```python
from build123d import *

# Parameters (mm, degrees)
SKETCH1_R           = 6.35
BOSS_EXTRUDE1_DEPTH = 15.875
SKETCH2_R           = 7.9375
BOSS_EXTRUDE2_DEPTH = 22.225
BOSS_EXTRUDE3_START = 69.85
SKETCH3_R           = 6.35
BOSS_EXTRUDE3_DEPTH = 69.85
SKETCH4_R           = 6.35
BOSS_EXTRUDE4_DEPTH = 47.625
SKETCH5_OUTSIDE_W   = 52.458
SKETCH5_OUTSIDE_H   = 52.458
SKETCH5_OUTSIDE_R   = 6.223
CUT_EXTRUDE3_DEPTH  = 19.05
SKETCH6_OUTSIDE_W   = 52.458
SKETCH6_OUTSIDE_H   = 52.458
SKETCH6_OUTSIDE_R   = 6.223
CUT_EXTRUDE4_DEPTH  = 19.05


with BuildPart() as part:
    # Sketch1 → Boss-Extrude1 (new, symmetric)
    with BuildSketch(Plane(origin=(0, 0, 0), x_dir=(0, 0, -1), z_dir=(1, 0, 0))):
        Circle(SKETCH1_R)
    extrude(amount=BOSS_EXTRUDE1_DEPTH, both=True)

    # Sketch2 → Boss-Extrude2 (add)
    with BuildSketch(Plane.ZY.offset(15.875)):
        Circle(SKETCH2_R)
    extrude(amount=BOSS_EXTRUDE2_DEPTH)

    # Sketch3 → Boss-Extrude3 (add)
    with BuildSketch(Plane(origin=(15.875, 0, 0), x_dir=(0, 0, -1), z_dir=(1, 0, 0)).offset(BOSS_EXTRUDE3_START)):
        with Locations(Location((0, 0, 0), (0, 0, 180))):
            Circle(SKETCH3_R)
    extrude(amount=-BOSS_EXTRUDE3_DEPTH)

    # Sketch4 → Boss-Extrude4 (add)
    with BuildSketch(Plane.ZY.offset(38.1)):
        Circle(SKETCH4_R)
    extrude(amount=BOSS_EXTRUDE4_DEPTH)

    # Sketch5 outside → Cut-Extrude3 (cut)
    with BuildSketch(Plane.ZY.offset(85.725)):
        Rectangle(SKETCH5_OUTSIDE_W, SKETCH5_OUTSIDE_H)
        Circle(SKETCH5_OUTSIDE_R, mode=Mode.SUBTRACT)
    extrude(amount=-CUT_EXTRUDE3_DEPTH, mode=Mode.SUBTRACT)

    # Sketch6 outside → Cut-Extrude4 (cut)
    with BuildSketch(Plane(origin=(85.725, 0, 0), x_dir=(0, 0, -1), z_dir=(1, 0, 0))):
        Rectangle(SKETCH6_OUTSIDE_W, SKETCH6_OUTSIDE_H)
        with Locations(Location((0, 0, 0), (0, 0, 180))):
            Circle(SKETCH6_OUTSIDE_R, mode=Mode.SUBTRACT)
    extrude(amount=-CUT_EXTRUDE4_DEPTH, mode=Mode.SUBTRACT)


solid = part.part
```
Check sheet for the modelled part. Datum: model origin and axes. Units: mm. A direction names the side the tool comes from. Coordinates: 2 decimals unless noted, no trailing zeros. Loops run counter-clockwise (first coordinate to the right, second up) from the corner with the lowest first, then second, coordinate; pieces in that order, holes last.
1) Gauge pin test, flat ends, axial feed: pin 1 (6 mm diameter, centred on x = 20.5, y = 6, fed in from +Z); pin 2 (1 mm diameter, centred on x = -14, z = -2.5, fed in from -Y); pin 3 (1 mm diameter, centred on x = -41, z = 0.5, fed in from -Y). Record the tip position at first contact, or that the pin passes through.
2) Access from +Z, -Z, +X, -X, +Y, -Y to the whole of each face (thin tool, end or side, straight path). Record for faces 1 (the face through (-76.333, -6.075, -1.349)), 2 (the face through (-15.875, 7, 0)), 3 (the face through (85.725, 0, 0)).
3) Sectioned sample at C-C (x = 40.5). Record the boundary of the cut face in (y, z).
4) Material ranges on probe 1 along Z at (x, y) = (3.5, 1.25); probe 2 along Y at (x, z) = (24, 0.5); probe 3 along X at (y, z) = (-2.5, 7.25) (3 decimals), recorded low to high.
Check sheet entries:
1. pin 1: stops at z = 5.6
1. pin 2: stops at y = -6.03
1. pin 3: stops at y = -6.35
2. face 1: -X
2. face 2: +X
2. face 3: +Z, -Z, +X, +Y, -Y
3. outline: circle Ø12.7 at (0, 0)
4. probe 1: z = -6.23 to 6.23
4. probe 2: y = -6.33 to 6.33
4. probe 3: x = -38.1 to -15.875
